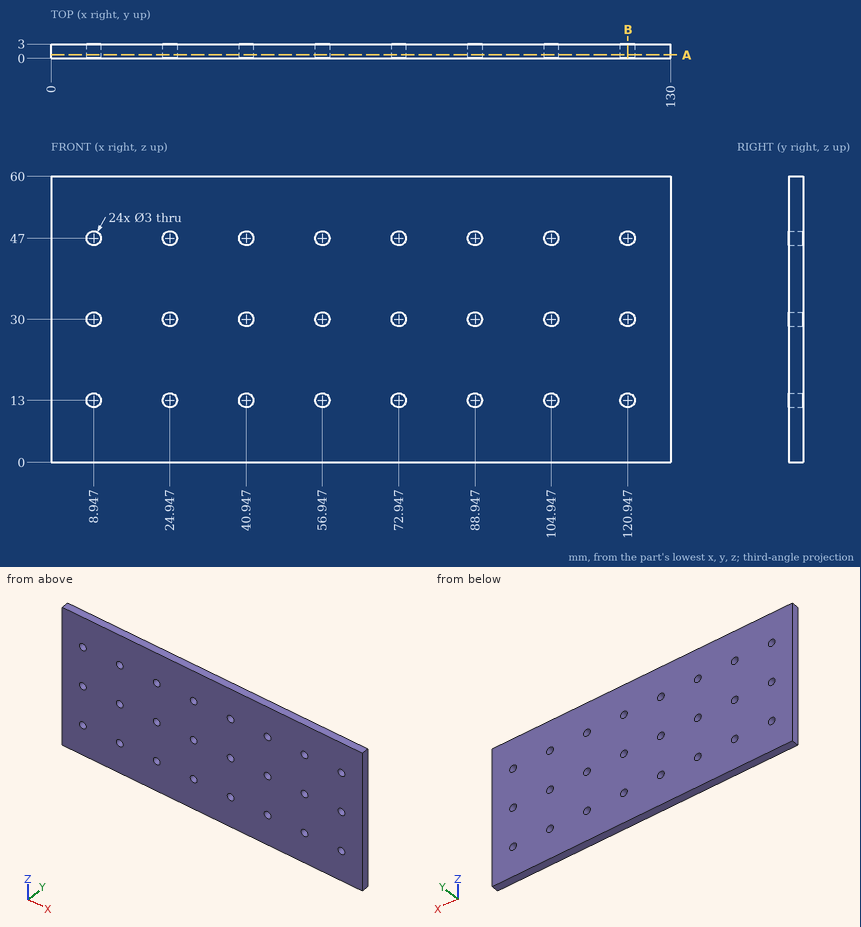
Geometry: see drawing. Coordinates: mm, zero at the bounding-box minimum. Give positions to 0.01 mm unless a question says otherwise; leave off trailing zeros. Order: outer loops, then holes, each group sorted by start corner. A loop starts at its lowest first (then second) coordinate and runs counter-clockwise, first axis right, second up. Notation, with made-up numbers: M -12.75,7.5 L 0.25,7.5 A6 cw 0.25,14.5 Z; hole C -13,43 d2. An arc over 180 degrees is marked long. Answer as CSV lines item,"result". Start each with the question number.
1) Line query: line 1 (Z direction, x = 40.5, y = 1.7); line 2 (Z direction, x = 26, y = 1). Output: solid intervals per line, ascending. Write a range as from..to.
2) Cut plane B-B (x = 121). Output: boundary loops of the cut face in (y, z), then the cut area to 3 significant figures.
3) Cut plane A-A (y = 0.7). State how many separate pieces and enclosed holes the cut face has, then the cut area to 3 significant figures.
Findings below:
1,line 1,"z = 0..11.57, 14.43..28.57, 31.43..45.57, 48.43..60"
1,line 2,"z = 0..11.93, 14.07..28.93, 31.07..45.93, 48.07..60"
2,outline,"M 0,0 L 3,0 L 3,11.5 L 0,11.5 Z; M 0,14.5 L 3,14.5 L 3,28.5 L 0,28.5 Z; M 0,31.5 L 3,31.5 L 3,45.5 L 0,45.5 Z; M 0,48.5 L 3,48.5 L 3,60 L 0,60 Z"
2,area,"153 mm²"
3,separate pieces,"1"
3,enclosed holes,"24"
3,area,"7,630 mm²"
